Read the model definition and answer for the solid it produces. Units are mm, in the model's axes. A direction names the side the tool comes from. Coordinates: 2 decimals unless noted, no trailing zeros. Write each loop counter-clockwise with the first axis right and the second up, starting at its lowest first coordinate (ties: lowest second). Pieces come first, ordered by that corner, then holes.
(1) Section D-D on z = 1.2 is taken. Write down the section's boundary in (x, y).
(2) Find the intervals of material crossed by probe 1 along X at (y, z) = (-1.75, 3); probe 2 along X at (y, z) = (0.25, 2.75); probe 3 along X at (y, z) = (1, 0.5), in increasing order.
(3) The mould has two halves that part along Y. Classify faces 3 (the cylindrical face through (-36.224, -7.18, 2.859)), 4 (the flat face through (-26, -3, 3.2)), 5 (the flat face through (-25, -8, 0)): +Y half, -Y half, draft (parallel to the pull), parting line (faces both ways), or undercut.
(4) Given pin 1 (1.5 mm diameter, centred on y = -0.5, z = 1, fed in from -X); pin 2 (5 mm diameter, centred on x = -28.5, y = -3, fed in from -Z); pin 3 (2 mm diameter, centred on x = -31, z = 0.5, fed in from -Y), each flat-ended and moving along its own axis, determine where each tip first touches the part or whether it passes through.
(5) Section C-C on y = -2.5 is taken. Write down the section's boundary in (x, z).
(6) Which of the six approach directions +Z, -Z, +X, -X, +Y, -Y give full straight-line access (tool end or side, diameter ignored) to faces 1 (the cylindrical face through (-22.69, -1.42, 1.58)), 2 (the cylindrical face through (-27.684, -1.642, 2.961))?
(7) Section B-B on x = -32 is taken. Write down the section's boundary in (y, z).
(8) Section A-A on y = 0.5 is taken. Write down the section's boundary in (x, z).
from build123d import *

# Parameters (mm, degrees)
SKETCH1_R           = 9
BOSS_EXTRUDE1_DEPTH = 5.8
SKETCH2_R           = 6.4
CUT_EXTRUDE1_DEPTH  = 3.2
SKETCH3_R           = 1
BOSS_EXTRUDE2_DEPTH = 3
SKETCH4_R           = 3.15
BOSS_EXTRUDE3_DEPTH = 3
SKETCH5_R           = 1.4
CUT_EXTRUDE2_DEPTH  = 40.9523428


with BuildPart() as part:
    # Sketch1 → Boss-Extrude1 (new body)
    with BuildSketch(Plane.XY):
        with Locations((-29.082250471, -1.703826149)):
            Circle(SKETCH1_R)
    extrude(amount=BOSS_EXTRUDE1_DEPTH)

    # Sketch2 → Cut-Extrude1 (cut)
    with BuildSketch(Plane(origin=(0, 0, 0), x_dir=(-1, 0, 0), z_dir=(0, 0, -1))):
        with Locations((29.082250471, -1.703826149)):
            Circle(SKETCH2_R)
    extrude(amount=-CUT_EXTRUDE1_DEPTH, mode=Mode.SUBTRACT)

    # Sketch3 → Boss-Extrude2 (add)
    with BuildSketch(Plane(origin=(0, 0, 3.2), x_dir=(-1, 0, 0), z_dir=(0, 0, -1))):
        with Locations((29.082250471, -1.703826149)):
            Circle(SKETCH3_R)
    extrude(amount=BOSS_EXTRUDE2_DEPTH)

    # Sketch4 → Boss-Extrude3 (add)
    with BuildSketch(Plane(origin=(0, 0, 0.2), x_dir=(-1, 0, 0), z_dir=(0, 0, -1))):
        with Locations((29.082250471, -1.703826149)):
            Circle(SKETCH4_R)
    extrude(amount=-BOSS_EXTRUDE3_DEPTH)

    # Sketch5 → Cut-Extrude2 (cut, through all)
    with BuildSketch(Plane(origin=(0, 0, 0.2), x_dir=(-1, 0, 0), z_dir=(0, 0, -1))):
        with Locations((29.082250471, -1.703826149)):
            Circle(SKETCH5_R)
    extrude(amount=-CUT_EXTRUDE2_DEPTH, mode=Mode.SUBTRACT)


solid = part.part
Response:
1. outline: circle Ø18 at (-29.08, -1.7); circle Ø6.3 at (-29.08, -1.7); hole circle Ø12.8 at (-29.08, -1.7); hole circle Ø2.8 at (-29.08, -1.7)
2. probe 1: x = -38.08 to -35.48, -32.23 to -30.48, -27.68 to -25.93, -22.68 to -20.08
2. probe 2: x = -37.87 to -35.18, -31.55 to -26.61, -22.99 to -20.3
2. probe 3: x = -37.67 to -34.88, -30.7 to -27.47, -23.28 to -20.5
3. face 3: parting line
3. face 4: undercut
3. face 5: draft
4. pin 1: stops at x = -38.07
4. pin 2: stops at z = 0.2
4. pin 3: stops at y = -10.66
5. outline: (-38.05, 0) - (-35.43, 0) - (-35.43, 3.2) - (-32.13, 3.2) - (-32.13, 0.2) - (-30.23, 0.2) - (-30.23, 5.8) - (-38.05, 5.8) - close; (-27.93, 0.2) - (-26.03, 0.2) - (-26.03, 3.2) - (-22.73, 3.2) - (-22.73, 0) - (-20.12, 0) - (-20.12, 5.8) - (-27.93, 5.8) - close
6. face 1: -Z
6. face 2: +Z, -Z
7. outline: (-10.22, 0) - (-7.4, 0) - (-7.4, 3.2) - (-2.89, 3.2) - (-2.89, 0.2) - (-0.52, 0.2) - (-0.52, 3.2) - (3.99, 3.2) - (3.99, 0) - (6.81, 0) - (6.81, 5.8) - (-10.22, 5.8) - close
8. outline: (-37.81, 0) - (-35.09, 0) - (-35.09, 3.2) - (-31.33, 3.2) - (-31.33, 0.2) - (-26.83, 0.2) - (-26.83, 3.2) - (-23.07, 3.2) - (-23.07, 0) - (-20.36, 0) - (-20.36, 5.8) - (-37.81, 5.8) - close
